CAD build for the part. Positions are in the model's coordinates, mm. A direction names the side the tool comes from. Give positions to 0.01 mm unless a question says otherwise; leave off trailing zeros. Order: outer loops, then holes, each group sorted by start corner. A loop starts at its lowest first (then second) coordinate and runs counter-clockwise, first axis right, second up.
Autodesk Inventor part; units mm, degrees
ref_plane "YZ Plane" through (0, 0, 0) normal (1, 0, 0) x (0, 1, 0)
ref_plane "XZ Plane" through (0, 0, 0) normal (0, 1, 0) x (-1, 0, 0)
ref_plane "XY Plane" through (0, 0, 0) normal (0, 0, 1) x (1, 0, 0)
sketch "Sketch1" plane through (0, 0, 0) normal (0, 0, 1) x (1, 0, 0)
  line L0 (-201.9864, -0.0159) -> (-218.1154, -0.0159) construction
  line L1 (-201.9864, -68.5959) -> (-218.1154, -68.5959) construction
  circle A0 centre (-234.0413, -9.3123) radius 2.5 construction
  circle A1 centre (-234.0413, -34.3059) radius 2.5 construction
  circle A2 centre (-234.0413, -59.2995) radius 2.5 construction
  line L2 (0.4039, -68.5877) -> (16.5329, -68.5877) construction
  line L3 (0.4039, -0.0077) -> (16.5329, -0.0077) construction
  circle A3 centre (27.9587, -59.2913) radius 2.5 construction
  circle A4 centre (27.9587, -34.2977) radius 2.5 construction
  circle A5 centre (27.9587, -9.3041) radius 2.5 construction
  line L4 (-243.0413, -0.0159) -> (36.9587, -0.0159)
  line L5 (36.9587, -0.0159) -> (36.9587, -68.5959)
  line L6 (36.9587, -68.5959) -> (-243.0413, -68.5959)
  line L7 (-243.0413, -68.5959) -> (-243.0413, -0.0159)
  line L8 (-103.0413, -534.726) -> (-103.0413, 430.7972) construction
  point P0 (0, 0)
  dimension "w" = 280
  dimension "d23" = 140
  dimension "d" = 262
  dimension "d34" = 131
extrude "Extrusion1" add sketch "Sketch1" along normal blind 12
sketch "Sketch4" plane through (0, 0, 0) normal (0, 0, -1) x (-1, 0, 0)
  circle A0 centre (65.5413, -59.3059) radius 2.5 construction
  circle A1 centre (40.5413, -59.3059) radius 2.5 construction
  circle A2 centre (140.5413, -9.3059) radius 2.5 construction
  circle A3 centre (115.5413, -9.3059) radius 2.5 construction
  line L0 (40.5413, -59.3059) -> (172.5963, -59.3059) construction
  line L1 (167.5124, -9.3059) -> (3.0086, -9.3059) construction
  line L2 (243.0413, -0.0159) -> (-36.9587, -0.0159) construction
  line L3 (38.0413, -9.3059) -> (168.0413, -9.3059) construction
  line L4 (38.0413, -12.3559) -> (168.0413, -12.3559)
  line L5 (168.0413, -6.2559) -> (38.0413, -6.2559)
  arc A4 (38.0413, -6.2559) -> (38.0413, -12.3559) centre (38.0413, -9.3059) ccw
  arc A5 (168.0413, -12.3559) -> (168.0413, -6.2559) centre (168.0413, -9.3059) ccw
  line L6 (103.0413, 455.7975) -> (103.0413, -509.7257) construction
  line L7 (38.0413, -59.3059) -> (168.0413, -59.3059) construction
  line L8 (38.0413, -62.3559) -> (168.0413, -62.3559)
  line L9 (168.0413, -56.2559) -> (38.0413, -56.2559)
  arc A6 (38.0413, -56.2559) -> (38.0413, -62.3559) centre (38.0413, -59.3059) ccw
  arc A7 (168.0413, -62.3559) -> (168.0413, -56.2559) centre (168.0413, -59.3059) ccw
  point P0 (0, 0)
  point P1 (-36.9587, -0.0159)
  point P2 (103.0413, -9.3059)
  point P3 (103.0413, -59.3059)
  dimension "d10" = 9.29
  dimension "d11" = 6.1
  dimension "d12" = 65
  dimension "d13" = 65
  dimension "d14" = 6.1
  dimension "d15" = 65
  dimension "d16" = 65
extrude "Extrusion2" cut sketch "Sketch4" against normal blind 12
sketch "Sketch5" plane through (0, 0, 0) normal (0, 0, -1) x (-1, 0, 0)
  line L0 (45.6373, -31.0674) -> (77.6413, -31.0674) construction
  arc A0 (168.0413, -12.3559) -> (168.0413, -6.2559) centre (168.0413, -9.3059) ccw construction
  arc A1 (168.0413, -62.3559) -> (168.0413, -56.2559) centre (168.0413, -59.3059) ccw construction
  arc A2 (38.0413, -6.2559) -> (38.0413, -12.3559) centre (38.0413, -9.3059) ccw construction
  arc A3 (38.0413, -56.2559) -> (38.0413, -62.3559) centre (38.0413, -59.3059) ccw construction
  line L1 (38.0413, -9.3059) -> (168.0413, -9.3059) construction
  line L2 (-36.9587, -0.0159) -> (243.0413, -0.0159)
  line L3 (38.0413, -14.5559) -> (168.0413, -14.5559)
  line L4 (168.0413, -4.0559) -> (38.0413, -4.0559)
  arc A4 (38.0413, -4.0559) -> (38.0413, -14.5559) centre (38.0413, -9.3059) ccw
  arc A5 (168.0413, -14.5559) -> (168.0413, -4.0559) centre (168.0413, -9.3059) ccw
  line L5 (38.0413, -59.3059) -> (168.0413, -59.3059) construction
  line L6 (38.0413, -64.5559) -> (168.0413, -64.5559)
  line L7 (168.0413, -54.0559) -> (38.0413, -54.0559)
  arc A6 (38.0413, -54.0559) -> (38.0413, -64.5559) centre (38.0413, -59.3059) ccw
  arc A7 (168.0413, -64.5559) -> (168.0413, -54.0559) centre (168.0413, -59.3059) ccw
  point P0 (0, 0)
  point P1 (243.0413, -0.0159)
  point P2 (103.0413, -9.3059)
  point P3 (103.0413, -59.3059)
  dimension "d19" = 10.5
  dimension "d20" = 10.5
extrude "Extrusion3" cut sketch "Sketch5" against normal blind 6.5
sketch "Sketch6" plane through (0, 0, 12) normal (0, 0, 1) x (1, 0, 0)
  line L0 (-103.0413, -534.726) -> (-103.0413, 430.7972) construction
  point P0 (0, 0)
  point P1 (27.9587, -59.3064)
  point P2 (27.9587, -34.3064)
  point P3 (27.9587, -9.3064)
  point P4 (-234.0413, -59.3147)
  point P5 (-234.0413, -34.3147)
  point P6 (-234.0413, -9.3147)
  dimension "d36" = 25
  dimension "d37" = 262
  dimension "d38" = 131
hole "Hole2" at (27.9587, -59.3064, 12) at (27.9587, -34.3064, 12) at (27.9587, -9.3064, 12) at (-234.0413, -59.3147, 12) at (-234.0413, -34.3147, 12) at (-234.0413, -9.3147, 12) direction (0, 0, -1) diameter 6.1 end through all counterbore diameter 11.5 counterbore depth 7
equation "\"d23\" = 0.5 * w"
equation "\"d34\" = 0.5 * d"
properties part number "ASI_mesoSPIM_Bridge"
1. Saw through at B-B on y = -34. Give the cut face in (x, z), plus the area to 3 significant figures.
2. Saw through at C-C on z = 10. State how many separate pieces and enclosed holes the cut face has, plus the area to 3 significant figures.
3. Wall check: line 1 (Y direction, x = -134, z = 4.5); line 2 (X direction, y = -9, z = 8.5); line 3 (Y direction, x = -138, z = 8.25). Give the ranges that are in metal, low to high.
4. Mould opens along X. For faces 1 (the flat face through (-243.041, -35, 6)), 2 (the cylindrical face through (25.897, -57.058, 2.465)), 3 (the flat face through (-105, -34, 0)) say: released by +X, released by -X, zero draft, split by the parting line, or undercut.
5. Saw through at A-A on x = -98.5. Give the cut face in (y, z), plus the area to 3 significant figures.
6. Pin check, flat tips, straight feed: P1, Ø8, axis at x = 27.96, y = -9.31, coming from the +Z side; P2, Ø5.5, axis at x = 27.96, y = -34.31, coming from the +Z side. Stop position of each tip, or through.
7. 3-axis set-ups, long thin cutter, end or side, ignore diameter. For faces 4 (the flat face through (30, -37, 5)), 5 (the cylindrical face through (-32.793, -9.19, 3.204)), 6 (the cylindrical face through (-34.992, -9.239, 9.212)): which of +Z, -Z, +X, -X, +Y, -Y reach the whole face in a straight line?
Reported:
1. outline: (-243.04, 0) - (-237.08, 0) - (-237.08, 5) - (-239.78, 5) - (-239.78, 12) - (-243.04, 12) - close; (-231.01, 0) - (24.92, 0) - (24.92, 5) - (22.22, 5) - (22.22, 12) - (-228.3, 12) - (-228.3, 5) - (-231.01, 5) - close; (30.99, 0) - (36.96, 0) - (36.96, 12) - (33.7, 12) - (33.7, 5) - (30.99, 5) - close
1. area: 3,140 mm2
2. separate pieces: 1
2. enclosed holes: 8
2. area: 16,900 mm2
3. line 1: y = -68.6 to -64.56, -54.06 to -14.56, -4.06 to -0.02
3. line 2: x = -243.04 to -239.78, -228.3 to -171.08, -35.01 to 22.22, 33.7 to 36.96
3. line 3: y = -68.6 to -62.36, -56.26 to -12.36, -6.26 to -0.02
4. face 1: released by -X
4. face 2: undercut
4. face 3: zero draft
5. outline: (-68.6, 0) - (-64.56, 0) - (-64.56, 6.5) - (-62.36, 6.5) - (-62.36, 12) - (-68.6, 12) - close; (-56.26, 6.5) - (-54.06, 6.5) - (-54.06, 0) - (-14.56, 0) - (-14.56, 6.5) - (-12.36, 6.5) - (-12.36, 12) - (-56.26, 12) - close; (-6.26, 6.5) - (-4.06, 6.5) - (-4.06, 0) - (-0.02, 0) - (-0.02, 12) - (-6.26, 12) - close
5. area: 619 mm2
6. P1: stops at z = 5
6. P2: passes through
7. face 4: +Z
7. face 5: -Z
7. face 6: +Z, -Z
